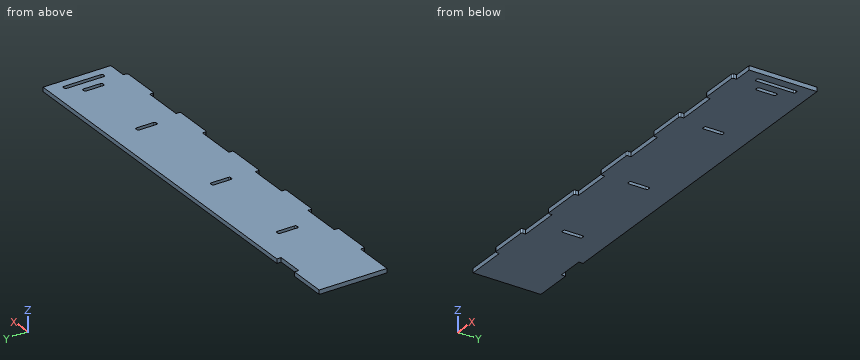
from build123d import *

# Parameters (mm, degrees)
SKETCH1_W           = 314.33
SKETCH1_H           = 50.8
BOSS_EXTRUDE1_DEPTH = 3.175
SKETCH2_W           = 3.175
SKETCH2_H           = 15
CUT_EXTRUDE1_DEPTH  = 4.175
SKETCH3_W           = 30
SKETCH3_H           = 3.175
BOSS_EXTRUDE2_DEPTH = 3.175
SKETCH4_W           = 3.175
SKETCH4_H           = 30
SKETCH4_H_2         = 15
CUT_EXTRUDE2_DEPTH  = 4.175
SKETCH5_W           = 20
SKETCH5_H           = 3.175
CUT_EXTRUDE3_DEPTH  = 4.175
FILLET1_R           = 1


with BuildPart() as part:
    # Sketch1 → Boss-Extrude1 (new body)
    with BuildSketch(Plane.XY):
        Rectangle(SKETCH1_W, SKETCH1_H)
    extrude(amount=BOSS_EXTRUDE1_DEPTH)

    # Sketch2 → Cut-Extrude1 (cut, through all)
    with BuildSketch(Plane.XY.offset(3.175)):
        with Locations((-80.9625, -0.9)):
            Rectangle(SKETCH2_W, SKETCH2_H)
        with Locations((-5.7375, -0.9)):
            Rectangle(SKETCH2_W, SKETCH2_H)
    extrude(amount=-CUT_EXTRUDE1_DEPTH, mode=Mode.SUBTRACT)

    # Sketch3 → Boss-Extrude2 (add)
    with BuildSketch(Plane.XZ.offset(25.4)):
        with Locations((-112.165, 1.5875)):
            Rectangle(SKETCH3_W, SKETCH3_H)
        with Locations((-52.165, 1.5875)):
            Rectangle(SKETCH3_W, SKETCH3_H)
        with Locations((127.835, 1.5875)):
            Rectangle(SKETCH3_W, SKETCH3_H)
        with Locations((67.835, 1.5875)):
            Rectangle(SKETCH3_W, SKETCH3_H)
        with Locations((7.835, 1.5875)):
            Rectangle(SKETCH3_W, SKETCH3_H)
    extrude(amount=BOSS_EXTRUDE2_DEPTH)

    # Sketch4 → Cut-Extrude2 (cut, through all)
    with BuildSketch(Plane.XY.offset(3.175)):
        with Locations((149.2275, 0)):
            Rectangle(SKETCH4_W, SKETCH4_H)
        with Locations((139.6975, -0.9)):
            Rectangle(SKETCH4_W, SKETCH4_H_2)
        with Locations((79.3725, -0.9)):
            Rectangle(SKETCH4_W, SKETCH4_H_2)
    extrude(amount=-CUT_EXTRUDE2_DEPTH, mode=Mode.SUBTRACT)

    # Sketch5 → Cut-Extrude3 (cut, through all)
    with BuildSketch(Plane.XY.offset(3.175)):
        with Locations((-119.065, 23.8125)):
            Rectangle(SKETCH5_W, SKETCH5_H)
    extrude(amount=-CUT_EXTRUDE3_DEPTH, mode=Mode.SUBTRACT)

    # Fillet1
    fillet1_edges = [part.edges().sort_by_distance(p)[0] for p in [
        (22.835, -28.575, 1.5875),
        (-7.165, -28.575, 1.5875),
        (147.64, -15, 1.5875),
        (147.64, 15, 1.5875),
        (150.815, 15, 1.5875),
        (150.815, -15, 1.5875),
        (141.285, 6.6, 1.5875),
        (141.285, -8.4, 1.5875),
        (138.11, -8.4, 1.5875),
        (138.11, 6.6, 1.5875),
        (80.96, 6.6, 1.5875),
        (80.96, -8.4, 1.5875),
        (77.785, -8.4, 1.5875),
        (77.785, 6.6, 1.5875),
        (-82.55, -8.4, 1.5875),
        (-82.55, 6.6, 1.5875),
        (-79.375, 6.6, 1.5875),
        (-79.375, -8.4, 1.5875),
        (-4.15, 6.6, 1.5875),
        (-4.15, -8.4, 1.5875),
        (-7.325, -8.4, 1.5875),
        (-7.325, 6.6, 1.5875),
        (-97.165, -28.575, 1.5875),
        (-127.165, -28.575, 1.5875),
        (-37.165, -28.575, 1.5875),
        (-67.165, -28.575, 1.5875),
        (142.835, -28.575, 1.5875),
        (112.835, -28.575, 1.5875),
        (82.835, -28.575, 1.5875),
        (52.835, -28.575, 1.5875),
    ]]
    fillet(fillet1_edges, radius=FILLET1_R)


solid = part.part
The listing builds one solid part. Answer for the finished solid, in the listing's coordinates (mm). Coordinates: 2 decimals unless noted, no trailing zeros. Write each loop counter-clockwise with the first axis right and the second up, starting at its lowest first coordinate (ties: lowest second). Pieces come first, ordered by that corner, then holes. Notation, with made-up numbers: M 13,8 L 25,8 A24 ccw 25,34 Z; hole C 18,9 d7. An arc over 180 degrees is marked long. Use one line per item in the form item = value.
Item 1: Find section B-B, the plane x = -87. Give the vertices of the cut face in (y, z) (3 decimals), plus the area to 3 significant figures.
Model answer:
outline = M -25.4,0 L 25.4,0 L 25.4,3.175 L -25.4,3.175 Z
area = 161 mm2
Item 2: Find the intervals of material crossed by probe 1 along X at (y, z) = (4, 2.95) (3 decimals); probe 2 along X at (y, z) = (-25.5, 0.6) (3 decimals); probe 3 along X at (y, z) = (7.5, 0.2) (3 decimals), in increasing order.
Model answer:
probe_1 = -157.165 to -82.55, -79.375 to -7.325, -4.15 to 77.785, 80.96 to 138.11, 141.285 to 147.64, 150.815 to 157.165
probe_2 = -127.165 to -97.165, -67.165 to -37.165, -7.165 to 22.835, 52.835 to 82.835, 112.835 to 142.835
probe_3 = -157.165 to 147.64, 150.815 to 157.165
Item 3: Given P1, Ø10, axis at x = -24, y = -1, coming from the -Z side; P2, Ø1.7, axis at y = -26.5, z = 1, coming from the -X side (3 decimals); P3, Ø1.3, axis at x = -81, z = 1, coming from the -Y side; P4, Ø1.1, axis at y = -26.5, z = 1.5, coming from the +X side (3 decimals), each flat-ended and moving along its own axis, determine where each tip first touches the part or whether it passes through.
Model answer:
P1 = 0
P2 = -127.165
P3 = -25.4
P4 = 142.835
Item 4: Find section A-A, the plane z = 2.05. Give the number of separate pieces and of enclosed holes in the cut face, plus the area to 3 significant figures.
Model answer:
separate_pieces = 1
enclosed_holes = 5
area = 16,100 mm2
